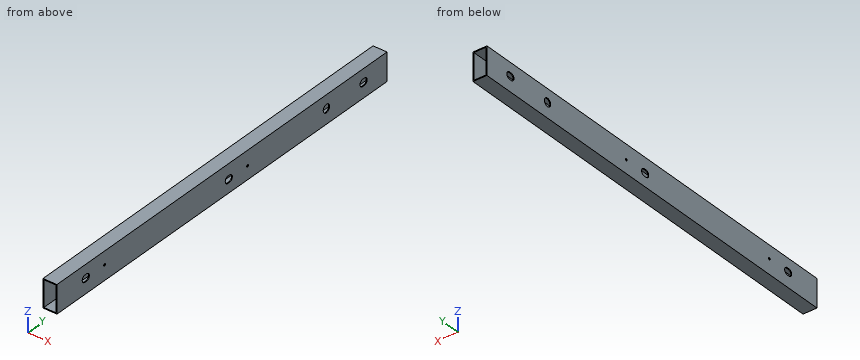
from build123d import *

# Parameters (mm, degrees)
F0_W     = 25.4
F0_H     = 50.8
F0_W_2   = 22.225
F0_H_2   = 47.625
F1_DEPTH = 762
F2_R     = 2.0066
F2_R_2   = 7.332348
F3_DEPTH = 25.401


with BuildPart() as f1:
    # F0 (on Front) → F1 (new body)
    with BuildSketch(Plane.XZ):
        with Locations((14.883514, 24.866902)):
            Rectangle(F0_W, F0_H)
        with Locations((14.883514, 24.866902)):
            Rectangle(F0_W_2, F0_H_2, mode=Mode.SUBTRACT)
    extrude(amount=F1_DEPTH)

    # F2 (on face) → F3 (cut, through all)
    with BuildSketch(Plane.YZ.offset(27.583514)):
        with BuildLine():
            Line((-697.333634, 20.167902), (-693.585719, 20.167902))
            ThreePointArc((-693.585719, 20.167902), (-687.235732, 26.505267), (-693.560449, 32.867852))
            ThreePointArc((-693.560449, 32.867852), (-693.585719, 32.867902), (-693.61099, 32.867852))
            Line((-693.61099, 32.867852), (-695.525434, 32.867852))
            ThreePointArc((-695.525434, 32.867852), (-695.550704, 32.867902), (-695.575975, 32.867852))
            Line((-695.575975, 32.867852), (-697.308364, 32.867852))
            ThreePointArc((-697.308364, 32.867852), (-697.333634, 32.867902), (-697.358904, 32.867852))
            ThreePointArc((-697.358904, 32.867852), (-701.832688, 30.999087), (-703.683634, 26.517902))
            ThreePointArc((-703.683634, 26.517902), (-701.823762, 22.027774), (-697.333634, 20.167902))
        make_face()
        with BuildLine():
            Line((-367.133634, 16.992902), (-363.385719, 16.992902))
            ThreePointArc((-363.385719, 16.992902), (-357.035732, 23.330267), (-363.360449, 29.692852))
            ThreePointArc((-363.360449, 29.692852), (-363.385719, 29.692902), (-363.41099, 29.692852))
            Line((-363.41099, 29.692852), (-365.325434, 29.692852))
            ThreePointArc((-365.325434, 29.692852), (-365.350704, 29.692902), (-365.375975, 29.692852))
            Line((-365.375975, 29.692852), (-367.108364, 29.692852))
            ThreePointArc((-367.108364, 29.692852), (-367.133634, 29.692902), (-367.158904, 29.692852))
            ThreePointArc((-367.158904, 29.692852), (-373.483621, 23.330267), (-367.133634, 16.992902))
        make_face()
        with BuildLine():
            Line((-55.999833, 20.167902), (-52.251919, 20.167902))
            ThreePointArc((-52.251919, 20.167902), (-45.901931, 26.505267), (-52.226648, 32.867852))
            ThreePointArc((-52.226648, 32.867852), (-52.251919, 32.867902), (-52.277189, 32.867852))
            Line((-52.277189, 32.867852), (-54.191633, 32.867852))
            ThreePointArc((-54.191633, 32.867852), (-54.216904, 32.867902), (-54.242174, 32.867852))
            Line((-54.242174, 32.867852), (-55.974563, 32.867852))
            ThreePointArc((-55.974563, 32.867852), (-55.999833, 32.867902), (-56.025104, 32.867852))
            ThreePointArc((-56.025104, 32.867852), (-62.349821, 26.505267), (-55.999833, 20.167902))
        make_face()
        with Locations((-321.866565, 23.342902)):
            Circle(F2_R)
        with Locations((-652.066565, 26.517902)):
            Circle(F2_R)
        with Locations((-139.925704, 26.517902)):
            Circle(F2_R_2)
    extrude(amount=-F3_DEPTH, mode=Mode.SUBTRACT)


solid = f1.part
Geometry: final body of the model. Coordinates: model frame, mm. Round coordinates to 2 decimals unless told otherwise and drop trailing zeros. Order: outer loops, then holes, each group sorted by start corner. A loop starts at its lowest first (then second) coordinate and runs counter-clockwise, first axis right, second up. Notation, with made-up numbers: (21.25, 3) -> (48.25, 3) arc R31 ccw to (48.25, 41) -> close; hole circle Ø10 at (85.5, 53.5). An arc over 180 degrees is marked (long way). Put each result on its own line as item: value. Start each with the question number.
Q1. Section C-C on y = -668.5. Return the cut outline in (x, z), and give its area (3 significant figures).
Q2. Section A-A on x = 7.75. Return the cut outline in (y, z).
Q3. Section B-B on z = 8.5. Return the cut outline in (x, y).
Q4. Line query: probe 1 along Z at (x, y) = (11.5, -228); probe 2 along X at (y, z) = (-337, 11). Output: solid intervals per line, ascending.
Ans:
1. outline: (2.18, -0.53) -> (27.58, -0.53) -> (27.58, 50.27) -> (2.18, 50.27) -> close; hole (3.77, 1.05) -> (26, 1.05) -> (26, 48.68) -> (3.77, 48.68) -> close
1. area: 232 mm2
2. outline: (-762, -0.53) -> (0, -0.53) -> (0, 1.05) -> (-762, 1.05) -> close; (-762, 48.68) -> (0, 48.68) -> (0, 50.27) -> (-762, 50.27) -> close
3. outline: (2.18, -762) -> (3.77, -762) -> (3.77, 0) -> (2.18, 0) -> close; (26, -762) -> (27.58, -762) -> (27.58, 0) -> (26, 0) -> close
4. probe 1: z = -0.53 to 1.05, 48.68 to 50.27
4. probe 2: x = 2.18 to 3.77, 26 to 27.58
